```python
from build123d import *

# Parameters (mm, degrees)
ENL_V_START             = -7
ESQUISSE2_R             = 1.5
ENL_V_MAT_EXTRU_1_DEPTH = 7


with BuildPart() as part:
    # Esquisse1 → Révolution1 (revolve)
    with BuildSketch(Plane.XY, mode=Mode.PRIVATE) as r_volution1_sk:
        Polygon((0, 0), (-14, 0), (-14, 7), (-12, 7), (-12, 2), (-10, 2), (-10, 11), (0, 11), align=None)
    revolve(r_volution1_sk.sketch.rotate(Axis((0, 0, 0), (0, 1, 0)), 270), axis=Axis((0, 0, 0), (0, 1, 0)))

    # Esquisse2 → Enlèv. mat.-Extru.1 (cut)
    with BuildSketch(Plane(origin=(0, 7, 0), x_dir=(1, 0, 0), z_dir=(0, 1, 0)).offset(ENL_V_START)):
        with Locations((14.848980609, 0)):
            Circle(ESQUISSE2_R)
        with Locations((14.382472578, -3.692791312)):
            Circle(ESQUISSE2_R)
        with Locations((13.012260899, -7.153550965)):
            Circle(ESQUISSE2_R)
        with Locations((10.824441013, -10.164826702)):
            Circle(ESQUISSE2_R)
        with Locations((7.956481688, -12.537408993)):
            Circle(ESQUISSE2_R)
        with Locations((4.588587357, -14.122219768)):
            Circle(ESQUISSE2_R)
        with Locations((0.932375207, -14.819679538)):
            Circle(ESQUISSE2_R)
        with Locations((-2.782421507, -14.585964338)):
            Circle(ESQUISSE2_R)
        with Locations((-6.322388444, -13.435759356)):
            Circle(ESQUISSE2_R)
        with Locations((-9.465096463, -11.441336201)):
            Circle(ESQUISSE2_R)
        with Locations((-12.013077662, -8.728011813)):
            Circle(ESQUISSE2_R)
        with Locations((-13.80623301, -5.466274344)):
            Circle(ESQUISSE2_R)
        with Locations((-14.731891962, -1.861070755)):
            Circle(ESQUISSE2_R)
        with Locations((-14.731891962, 1.861070755)):
            Circle(ESQUISSE2_R)
        with Locations((-13.80623301, 5.466274344)):
            Circle(ESQUISSE2_R)
        with Locations((-12.013077662, 8.728011813)):
            Circle(ESQUISSE2_R)
        with Locations((-9.465096463, 11.441336201)):
            Circle(ESQUISSE2_R)
        with Locations((-6.322388444, 13.435759356)):
            Circle(ESQUISSE2_R)
        with Locations((-2.782421507, 14.585964338)):
            Circle(ESQUISSE2_R)
        with Locations((0.932375207, 14.819679538)):
            Circle(ESQUISSE2_R)
        with Locations((4.588587357, 14.122219768)):
            Circle(ESQUISSE2_R)
        with Locations((7.956481688, 12.537408993)):
            Circle(ESQUISSE2_R)
        with Locations((10.824441013, 10.164826702)):
            Circle(ESQUISSE2_R)
        with Locations((13.012260899, 7.153550965)):
            Circle(ESQUISSE2_R)
        with Locations((14.382472578, 3.692791312)):
            Circle(ESQUISSE2_R)
    extrude(amount=ENL_V_MAT_EXTRU_1_DEPTH, mode=Mode.SUBTRACT)


solid = part.part
```
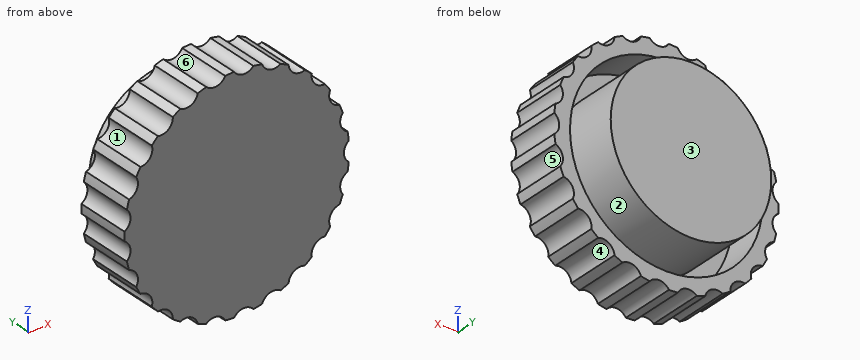
Source: CAD feature listing. Evaluate the final solid. Frame: model axes, mm. Face numbers are marked on the shaded views. A direction names the side the tool comes from. Round coordinates to 2 decimals unless told otherwise and drop trailing zeros. Loops run counter-clockwise (first coordinate to the right, second up) from the corner with the lowest first, then second, coordinate; pieces in that order, holes last. Notation, with made-up numbers: (45.5, -29) - (52.5, -29) arc R19 cw to (52.5, -7) - close; hole circle Ø8 at (15.5, 11). An arc over 180 degrees is marked (long way). Use CSV: the item, a comma, the result in double quotes.
Q1. Reachability of the marked faces 1 and 2 from +Z, -Z, +X, -X, +Y, -Y: full face, straight path, thin tool, end or side. Return the list, or none.
Reported:
face 1,"-X, +Y, -Y"
face 2,"+Y"
Q2. Ray query, line 1 along X through (y, z) = (3.75, 0); line 2 along X through (y, z) = (5, 3.5); line 3 along Z through (x, y) = (4.25, 6). Return the intervals inside material, ascending.
Reported:
line 1,"-14 to -12, -10 to 10, 12 to 13.35"
line 2,"-13.56 to -11.48, -9.37 to 9.37, 11.48 to 12.89"
line 3,"-12.66 to -11.22, -9.05 to 9.05, 11.22 to 12.66"
Q3. Mould query, pull axis Z, two halves, no side actions, for the marked faces 3, 4, 5 and 6. Classes: pulls with the +Z half, pulls with the -Z half, needs draft (parallel to the pull), parting line crosses it, or undercut.
Reported:
face 3,"needs draft"
face 4,"pulls with the -Z half"
face 5,"undercut"
face 6,"pulls with the +Z half"
Q4. Section query A-A, the plane y = 4.25. Give the number of separate pieces and of enclosed holes in the cut face, then the cut area to 3 significant figures.
Reported:
separate pieces,"2"
enclosed holes,"1"
area,"450 mm^2"
Q5. Pin query (flat end, axial travel): pin 1 Ø1 at (y, z) = (3, -10) entering from -X; pin 2 Ø5 at (x, y) = (5.5, 3) entering from -Z; pin 3 Ø5 at (x, y) = (2.5, 3.5) entering from +Z. Return the tip coordinate at first contact, or that it passes through.
Reported:
pin 1,"x = -10.28"
pin 2,"z = -13.67"
pin 3,"z = 13.85"
Q6. Section query C-C, the plane z = 0. Output: boundary loops of the cut face in (x, y), then the cut area to 3 significant figures.
Reported:
outline,"(-14, 0) - (13.35, 0) - (13.35, 7) - (12, 7) - (12, 2) - (10, 2) - (10, 11) - (-10, 11) - (-10, 2) - (-12, 2) - (-12, 7) - (-14, 7) - close"
area,"251 mm^2"
Q7. Section query D-D, the plane y = 9.75. Output: boundary loops of the cut face in (x, z).
Reported:
outline,"circle Ø20 at (0, 0)"
Q8. Section query B-B, the plane x = 0.5. Output: boundary loops of the cut face in (y, z), then the cut area to 3 significant figures.
Reported:
outline,"(0, -13.38) - (7, -13.38) - (7, -11.99) - (2, -11.99) - (2, -9.99) - (11, -9.99) - (11, 9.99) - (2, 9.99) - (2, 11.99) - (7, 11.99) - (7, 13.38) - (0, 13.38) - close"
area,"247 mm^2"
